Geometry check sheet. Reference: the model listing, model coordinates, mm. Round coordinates to 2 decimals unless told otherwise and drop trailing zeros. Order: outer loops, then holes, each group sorted by start corner. A loop starts at its lowest first (then second) coordinate and runs counter-clockwise, first axis right, second up. Notation, with made-up numbers: (22, -27.5) - (48, -27.5) arc R27 ccw to (48, 5.5) - close; hole circle Ø5 at (11, 37.25). An arc over 180 degrees is marked (long way). Return JSON: item names as keys, results as strings. Group by question number.
Q1. Sectioned sample at B-B, the plane z = 5.75. Record the cut outline in (x, y).
Q2. Sectioned sample at C-C, the plane x = 0. Record the cut outline in (y, z).
Q3. Sectioned sample at D-D, the plane z = 3. Record the cut outline in (x, y), then the cut area to 3 significant figures.
Q4. Gauge pin test, flat end, axial feed: pin 1 Ø2 at (y, z) = (-1, 2) entering from +X. Record the tip position at first contact, or that the pin passes through.
Q5. Draft check along Y on faces 1 (the cylindrical face through (2.192, -4.214, 3.168)), 2 (the cylindrical face through (-1.7, 0.32, 3.24)), 3 (the flat face through (0, 0, 0)). Enter one of: pulls with the +Y half, pulls with the -Y half, needs draft (parallel to the pull), parting line crosses it, or undercut.
Q6. Material ranges on line 1 along X through (y, z) = (-0.25, 5.25); line 2 along Y through (x, z) = (-2.25, 5.75); line 3 along Y through (x, z) = (-2, 1.5), recorded low to high.
Q7. Sectioned sample at A-A, the plane y = 0. Record the cut outline in (x, z).
```python
from build123d import *

# Parameters (mm, degrees)
F0_R     = 4.75
F1_DEPTH = 6.4
F2_R     = 1.05
F3_DEPTH = 6.401
F4_SIZE  = 0.9


with BuildPart() as f1:
    # F0 (on Top) → F1 (new body)
    with BuildSketch(Plane.XY):
        Circle(F0_R)
    extrude(amount=F1_DEPTH)

    # F2 (on face) → F3 (cut, through all)
    with BuildSketch(Plane.XY.offset(6.4)):
        with Locations((-2.7, 0)):
            Circle(F2_R)
    extrude(amount=-F3_DEPTH, mode=Mode.SUBTRACT)

    # F4
    f4_edges = [f1.edges().sort_by_distance(p)[0] for p in [
        (-4.75, 0, 6.4),
        (-4.75, 0, 0),
    ]]
    chamfer(f4_edges, length=F4_SIZE)


solid = f1.part
```
Reply:
{
 "1": {"outline": "circle Ø9 at (0, 0); hole circle Ø2.1 at (-2.7, 0)"},
 "2": {"outline": "(-4.75, 0.9) - (-3.85, 0) - (3.85, 0) - (4.75, 0.9) - (4.75, 5.5) - (3.85, 6.4) - (-3.85, 6.4) - (-4.75, 5.5) - close"},
 "3": {"outline": "circle Ø9.5 at (0, 0); hole circle Ø2.1 at (-2.7, 0)", "area": "67.4 mm^2"},
 "4": {"pin 1": "x = 4.75"},
 "5": {"face 1": "parting line crosses it", "face 2": "undercut", "face 3": "needs draft"},
 "6": {"line 1": "-4.74 to -3.72, -1.68 to 4.74", "line 2": "-3.9 to -0.95, 0.95 to 3.9", "line 3": "-4.31 to -0.78, 0.78 to 4.31"},
 "7": {"outline": "(-4.75, 0.9) - (-3.85, 0) - (-3.75, 0) - (-3.75, 6.4) - (-3.85, 6.4) - (-4.75, 5.5) - close; (-1.65, 0) - (3.85, 0) - (4.75, 0.9) - (4.75, 5.5) - (3.85, 6.4) - (-1.65, 6.4) - close"}
}
